The listing builds one solid part. Answer for the finished solid, in the listing's coordinates (mm). Face numbers are marked on the shaded views. A direction names the side the tool comes from. Coordinates: 2 decimals unless noted, no trailing zeros. Write each loop counter-clockwise with the first axis right and the second up, starting at its lowest first coordinate (ties: lowest second). Pieces come first, ordered by that corner, then holes.
(1) Which of the six approach directions +Z, -Z, +X, -X, +Y, -Y give full straight-line access (tool end or side, diameter ignored) to the marked faces 1, 2, 3, 4 and 5?
(2) Given P1, Ø9, axis at x = -58, y = 10, coming from the -Z side; P2, Ø9, axis at y = 13.5, z = 53.5, coming from the -X side; P3, Ø8, axis at y = 27, z = 13, coming from the -X side, each flat-ended and moving along its own axis, determine where each tip first touches the part or whether it passes through.
(3) The part is cut by section B-B on x = 0. Determine the outline of the cut face in (y, z).
(4) Straight lines are drawn through the part: line 1 (X direction, y = 4.5, z = 53); line 2 (Y direction, x = 7, z = 42). For each, find the intervals that lie inside material, in ascending order.
(5) The part is cut by section D-D on y = 38. Determine the outline of the cut face in (x, z), plus the area to 3 significant figures.
(6) The part is cut by section A-A on z = 0. Determine the outline of the cut face in (x, y), plus the area to 3 significant figures.
(7) The part is cut by section C-C on z = 55.5. Determine the outline of the cut face in (x, y).
(8) For a pull along Z with two mould halves and no side action, classify the marked faces 6, 7 and 8 as +Z half, -Z half, draft (parallel to the pull), parting line (faces both ways), or undercut.
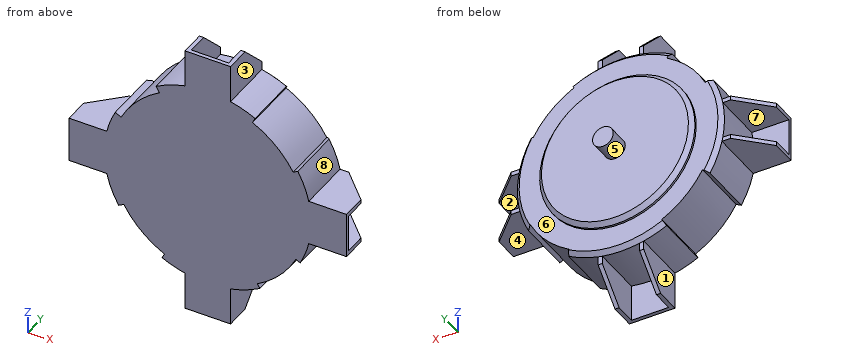
from build123d import *

# Parameters (mm, degrees)
SKETCH1_R           = 50
BOSS_EXTRUDE1_DEPTH = 28
SKETCH2_R           = 37.5
BOSS_EXTRUDE2_DEPTH = 3
CHAMFER1_SIZE       = 2
SKETCH3_R           = 5
BOSS_EXTRUDE3_DEPTH = 10
BOSS_EXTRUDE4_DEPTH = 67
CIRPATTERN6_COUNT   = 4
CHAMFER2_SIZE       = 14
CUT_EXTRUDE1_DEPTH  = 67
CIRPATTERN7_COUNT   = 4


with BuildPart() as part:
    # Sketch1 → Boss-Extrude1 (new body)
    with BuildSketch(Plane(origin=(0, 0, 0), x_dir=(1, 0, 0), z_dir=(0, 1, 0))):
        with Locations(Location((0, 0, 0), (0, 0, 270))):
            Circle(SKETCH1_R)
    extrude(amount=BOSS_EXTRUDE1_DEPTH)

    # Sketch2 → Boss-Extrude2 (add)
    with BuildSketch(Plane(origin=(0, 28, 0), x_dir=(1, 0, 0), z_dir=(0, 1, 0))):
        with Locations(Location((0, 0, 0), (0, 0, 270))):
            Circle(SKETCH2_R)
    extrude(amount=BOSS_EXTRUDE2_DEPTH)

    # Chamfer1
    chamfer1_edges = [part.edges().sort_by_distance(p)[0] for p in [
        (0, 28, -50),
        (0, 31, -37.5),
    ]]
    chamfer(chamfer1_edges, length=CHAMFER1_SIZE)

    # Sketch3 → Boss-Extrude3 (add)
    with BuildSketch(Plane(origin=(0, 31, 0), x_dir=(1, 0, 0), z_dir=(0, 1, 0))):
        with Locations(Location((0, 0, 0), (0, 0, 270))):
            Circle(SKETCH3_R)
    extrude(amount=BOSS_EXTRUDE3_DEPTH)

    # Sketch4 → Boss-Extrude4 (add)
    with BuildSketch(Plane.XY):
        Polygon((-8.998295996, 1.823065443), (8.998295996, 1.823065443), (8.998295996, 26), (10.998295996, 26), (10.998295996, 0), (-10.998295996, 0), (-10.998295996, 26), (-8.998295996, 26), align=None)
    boss_extrude4 = extrude(amount=-BOSS_EXTRUDE4_DEPTH)

    # CirPattern6: Boss-Extrude4 ×4 about axis
    cirpattern6_axis = Axis((0, 0, 0), (0, 1, 0))
    for i in range(1, CIRPATTERN6_COUNT):
        add(boss_extrude4.rotate(cirpattern6_axis, i * 360 / CIRPATTERN6_COUNT))

    # Chamfer2
    chamfer2_edges = [part.edges().sort_by_distance(p)[0] for p in [
        (9.998295996, 26, -67),
        (-9.998295996, 26, -67),
        (-67, 26, -9.998295996),
        (-9.998295996, 26, 67),
        (-67, 26, 9.998295996),
        (67, 26, 9.998295996),
        (67, 26, -9.998295996),
        (9.998295996, 26, 67),
    ]]
    chamfer(chamfer2_edges, length=CHAMFER2_SIZE)

    # Sketch10 → Cut-Extrude1 (cut)
    with BuildSketch(Plane(origin=(0, 0, 0), x_dir=(-1, 0, 0), z_dir=(0, -1, 0))):
        with BuildLine():
            Line((24.931942454, -43.340491985), (23.336298137, -40.566700498))
            ThreePointArc((23.336298137, -40.566700498), (34.044117933, -32.112895139), (41.858905353, -20.930170631))
            Line((41.858905353, -20.930170631), (44.721052728, -22.361293409))
            ThreePointArc((44.721052728, -22.361293409), (36.371920868, -34.308648652), (24.931942454, -43.340491985))
        make_face()
    cut_extrude1 = extrude(amount=-CUT_EXTRUDE1_DEPTH, mode=Mode.SUBTRACT)

    # CirPattern7: Cut-Extrude1 ×4 about axis
    cirpattern7_axis = Axis((0.338512389, 0, -0.319309576), (0, 1, 0))
    for i in range(1, CIRPATTERN7_COUNT):
        add(cut_extrude1.rotate(cirpattern7_axis, i * 360 / CIRPATTERN7_COUNT), mode=Mode.SUBTRACT)


solid = part.part
Model answer:
1. face 1: -Z, -X, +Y, -Y
1. face 2: +X, +Y
1. face 3: +Z, +X, +Y, -Y
1. face 4: -Z, +X, +Y, -Y
1. face 5: +Y
2. P1: stops at z = -11
2. P2: stops at x = -11
2. P3: stops at x = -55.46
3. outline: (0, -67) - (1.82, -67) - (1.82, -50) - (26, -50) - (28, -48) - (28, -37.5) - (29, -37.5) - (31, -35.5) - (31, -5) - (41, -5) - (41, 5) - (31, 5) - (31, 35.5) - (29, 37.5) - (28, 37.5) - (28, 48) - (26, 50) - (1.82, 50) - (1.82, 67) - (0, 67) - close
4. line 1: x = -11 to -9, 9 to 11
4. line 2: y = 0 to 28
5. outline: circle Ø10 at (0, 0)
5. area: 78.5 mm2
6. outline: (-67, 0) - (67, 0) - (67, 1.82) - (50, 1.82) - (50, 26) - (48, 28) - (37.5, 28) - (37.5, 29) - (35.5, 31) - (5, 31) - (5, 41) - (-5, 41) - (-5, 31) - (-35.5, 31) - (-37.5, 29) - (-37.5, 28) - (-48, 28) - (-50, 26) - (-50, 1.82) - (-67, 1.82) - close
6. area: 3,180 mm2
7. outline: (-11, 0) - (11, 0) - (11, 23.5) - (9, 23.5) - (9, 1.82) - (-9, 1.82) - (-9, 23.5) - (-11, 23.5) - close
8. face 6: draft
8. face 7: undercut
8. face 8: +Z half
